```python
from build123d import *

# Parameters (mm, degrees)
F0_W     = 747
F0_H     = 50
F0_R     = 4
F0_W_2   = 3
F1_DEPTH = 3
F2_DEPTH = 486
F3_W     = 750
F3_H     = 50
F3_R     = 4
F4_DEPTH = 3


with BuildPart() as f1:
    # F0 (on Right) → F1 (new body)
    with BuildSketch(Plane.YZ):
        with Locations((274.845328, 248.377842)):
            Rectangle(F0_W, F0_H)
        with Locations((-83.654672, 258.377842)):
            Circle(F0_R, mode=Mode.SUBTRACT)
        with Locations((316.345328, 258.377842)):
            Circle(F0_R, mode=Mode.SUBTRACT)
        with Locations((649.845328, 248.377842)):
            Rectangle(F0_W_2, F0_H)
    extrude(amount=F1_DEPTH)

    # F0 (on Right) → F2 (join)
    with BuildSketch(Plane.YZ):
        with Locations((649.845328, 248.377842)):
            Rectangle(F0_W_2, F0_H)
    extrude(amount=-F2_DEPTH)

    # F3 (on face) → F4 (join)
    with BuildSketch(Plane(origin=(-486, 0, 0), x_dir=(0, -1, 0), z_dir=(-1, 0, 0))):
        with Locations((-276.345328, 248.377842)):
            Rectangle(F3_W, F3_H)
        with Locations((-316.345328, 258.377842)):
            Circle(F3_R, mode=Mode.SUBTRACT)
        with Locations((83.654672, 258.377842)):
            Circle(F3_R, mode=Mode.SUBTRACT)
    extrude(amount=F4_DEPTH)


solid = f1.part
```
Model file for the job. Use its own axes, mm. A direction names the side the tool comes from. Coordinates: 2 decimals unless noted, no trailing zeros. Loops run counter-clockwise (first coordinate to the right, second up) from the corner with the lowest first, then second, coordinate; pieces in that order, holes last. Notation, with made-up numbers: (-11.5, -6) -> (32.5, -6) arc R26 cw to (32.5, 19) -> close; hole circle Ø9 at (86, -25). An arc over 180 degrees is marked (long way). Answer as a JSON object with one key per item and string values.
Q1. Cut at B-B (z = 243.5). List the corners of the cut face in (x, y).
Report:
{"outline": "(-489, -98.65) -> (-486, -98.65) -> (-486, 648.35) -> (0, 648.35) -> (0, -98.65) -> (3, -98.65) -> (3, 651.35) -> (-489, 651.35) -> close"}
Q2. 3-axis set-ups, long thin cutter, end or side, ignore diameter. For faces 1 (the flat face through (-240, 651.345, 248)), 2 (the flat face through (0, 270, 249)): which of +Z, -Z, +X, -X, +Y, -Y reach the whole face in a straight line?
Report:
{"face 1": "+Z, -Z, +X, -X, +Y", "face 2": "+Z, -Z, -Y"}
Q3. Cut at A-A (y = 541). List the corners of the cut face in (x, z), and give its area (3 significant figures).
Report:
{"outline": "(-489, 223.38) -> (-486, 223.38) -> (-486, 273.38) -> (-489, 273.38) -> close; (0, 223.38) -> (3, 223.38) -> (3, 273.38) -> (0, 273.38) -> close", "area": "300 mm2"}
Q4. Flat gauge pins, fed straight in: P1, Ø13, axis at y = 316.35, z = 258.38, coming from the +X side; P2, Ø15, axis at x = -145, z = 250.5, coming from the -Y side; P3, Ø7, axis at y = -83.65, z = 258.38, coming from the +X side. Where does each tip first touch, or does it go through?
Report:
{"P1": "stops at x = 3", "P2": "stops at y = 648.35", "P3": "passes through"}
Q5. Cut at C-C (x = -91.5). List the corners of the cut face in (y, z).
Report:
{"outline": "(648.35, 223.38) -> (651.35, 223.38) -> (651.35, 273.38) -> (648.35, 273.38) -> close"}
Q6. Pull direction X, two halves, no side cores. Call faces 3 (the flat face through (-240, 648.345, 248)), 4 (the flat face through (-489, 282, 249)), 5 (the flat face through (3, 271, 249)): released by +X, released by -X, zero draft, split by the parting line, or undercut.
Report:
{"face 3": "undercut", "face 4": "released by -X", "face 5": "released by +X"}
Q7. Probe probe 1 along X at (y, z) = (194, 263); probe 2 along Y at (x, z) = (-313, 270). List the from-to ranges inside material, lowest first.
Report:
{"probe 1": "x = -489 to -486, 0 to 3", "probe 2": "y = 648.35 to 651.35"}
